Could you check a few things on this model? Use its own coordinates, in mm. Coordinates: 2 decimals unless noted, no trailing zeros. Write each loop counter-clockwise with the first axis right and the second up, starting at its lowest first coordinate (ties: lowest second). Pieces come first, ordered by that corner, then holes.
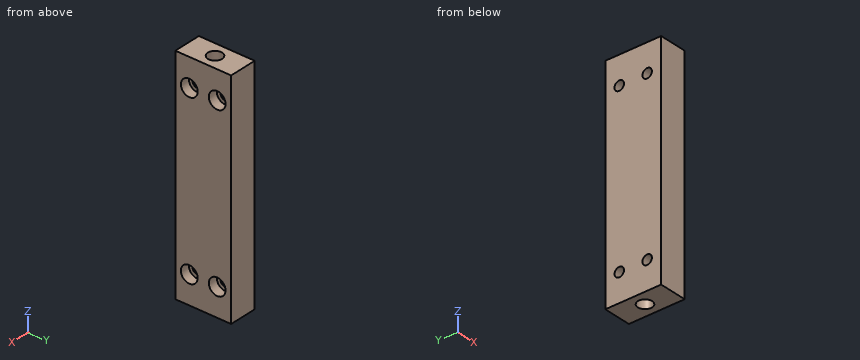
Autodesk Inventor part; units mm, degrees
ref_plane "YZ Plane" through (0, 0, 0) normal (1, 0, 0) x (0, 1, 0)
ref_plane "XZ Plane" through (0, 0, 0) normal (0, 1, 0) x (-1, 0, 0)
ref_plane "XY Plane" through (0, 0, 0) normal (0, 0, 1) x (1, 0, 0)
sketch "Sketch1" plane through (0, 0, 0) normal (0, 0, 1) x (1, 0, 0)
  line L0 (-13.202, 13.202) -> (-0.502, 13.202)
  line L1 (-0.502, 13.202) -> (-0.502, -12.198)
  line L2 (-0.502, -12.198) -> (-13.202, -12.198)
  line L3 (-13.202, -12.198) -> (-13.202, 13.202)
  point P0 (0, 0)
  dimension "d0" = 12.7
  dimension "d1" = 25.4
extrude "Extrusion1" add sketch "Sketch1" along normal blind 101.6
sketch "Sketch6" plane through (-0.502, 13.202, 101.6) normal (1, 0, 0) x (0, 0, -1)
  line L0 (101.6, 0) -> (101.6, -25.4)
  line L1 (101.6, -25.4) -> (0, -25.4)
  line L2 (101.6, 0) -> (101.6, -25.4)
  line L3 (101.6, 0) -> (0, 0)
  line L4 (0, -25.4) -> (0, 0)
  line L5 (0, -25.4) -> (0, 0)
  point P0 (101.6, -13.202)
  point P1 (88.9, -6.35)
  point P2 (88.9, -19.05)
  point P3 (101.6, -19.05)
  point P4 (101.6, -6.35)
  point P5 (12.7, -6.35)
  point P6 (12.7, -19.05)
  point P7 (0, -19.05)
  point P8 (0, -6.35)
  dimension "d51" = 12.7
  dimension "d52" = 6.35
  dimension "d53" = 12.7
  dimension "d54" = 6.35
  dimension "d55" = 12.7
  dimension "d56" = 6.35
  dimension "d57" = 12.7
  dimension "d58" = 6.35
sketch "Sketch8" plane through (0, 0, 101.6) normal (0, 0, 1) x (1, 0, 0)
  line L0 (-13.202, 13.202) -> (-13.202, -12.198)
  line L1 (-13.202, -12.198) -> (-0.502, -12.198)
  point P0 (0, 0)
  point P1 (-6.852, 0.502)
  dimension "d82" = 6.35
  dimension "d84" = 12.7
hole "Hole4" at (-6.852, 0.502, 101.6) direction (0, 0, -1) diameter 6.477 end through all
hole "Hole5" at (-0.502, 6.852, 12.7) at (-0.502, -5.848, 12.7) at (-0.502, 6.852, 88.9) at (-0.502, -5.848, 88.9) direction (-1, 0, 0) diameter 4.318 end through all counterbore diameter 7.62 counterbore depth 4.318
properties part number "BottomOfElevatorFrameMid"
Item 1: Will these pins go through, and if not, where does the flat tip stop? pin 1 Ø4 at (y, z) = (-5.848, 88.9) entering from -X; pin 2 Ø7 at (y, z) = (6.852, 88.9) entering from +X.
Item 2: I want a section at A-A, the plane z = 12.7. List the corners of the cut face in (x, y) for me.
Item 3: I want a section at B-B, the plane x = -2.25. List the corners of the cut face in (y, z) for me, then the cut area to 3 significant figures.
Item 4: If I drill on line 1 along Y through (x, z) = (-2.3, 88.9); line 2 along Z through (x, y) = (-4.75, 10); line 3 along Z through (x, y) = (-3, 9), over which ranges is the centre line in solid material (lowest first)?
Item 5: I want a section at D-D, the plane z = 64. List the corners of the cut face in (x, y) for me, then the cut area to 3 significant figures.
Item 6: I want a section at C-C, the plane y = -4.75. List the corners of the cut face in (x, z) for me, then the cut area to 3 significant figures.
Taken from the geometry:
1. pin 1: passes through
1. pin 2: stops at x = -4.82
2. outline: (-13.2, -12.2) - (-0.5, -12.2) - (-0.5, -9.66) - (-4.82, -9.66) - (-4.82, -8.01) - (-13.2, -8.01) - close; (-13.2, -3.69) - (-4.82, -3.69) - (-4.82, -2.04) - (-0.5, -2.04) - (-0.5, 3.04) - (-4.82, 3.04) - (-4.82, 4.69) - (-13.2, 4.69) - close; (-13.2, 9.01) - (-4.82, 9.01) - (-4.82, 10.66) - (-0.5, 10.66) - (-0.5, 13.2) - (-13.2, 13.2) - close; hole circle Ø6.48 at (-6.85, 0.5)
3. outline: (-12.2, 0) - (13.2, 0) - (13.2, 101.6) - (-12.2, 101.6) - close; hole circle Ø7.62 at (-5.85, 12.7); hole circle Ø7.62 at (-5.85, 88.9); hole circle Ø7.62 at (6.85, 12.7); hole circle Ø7.62 at (6.85, 88.9)
3. area: 2,400 mm2
4. line 1: y = -12.2 to -9.66, -2.04 to 3.04, 10.66 to 13.2
4. line 2: z = 0 to 10.55, 14.85 to 86.75, 91.05 to 101.6
4. line 3: z = 0 to 9.55, 15.85 to 85.75, 92.05 to 101.6
5. outline: (-13.2, -12.2) - (-0.5, -12.2) - (-0.5, 13.2) - (-13.2, 13.2) - close; hole circle Ø6.48 at (-6.85, 0.5)
5. area: 290 mm2
6. outline: (-13.2, 0) - (-0.5, 0) - (-0.5, 9.05) - (-4.82, 9.05) - (-4.82, 10.84) - (-13.2, 10.84) - close; (-13.2, 14.56) - (-4.82, 14.56) - (-4.82, 16.35) - (-0.5, 16.35) - (-0.5, 85.25) - (-4.82, 85.25) - (-4.82, 87.04) - (-13.2, 87.04) - close; (-13.2, 90.76) - (-4.82, 90.76) - (-4.82, 92.55) - (-0.5, 92.55) - (-0.5, 101.6) - (-13.2, 101.6) - close
6. area: 1,160 mm2
